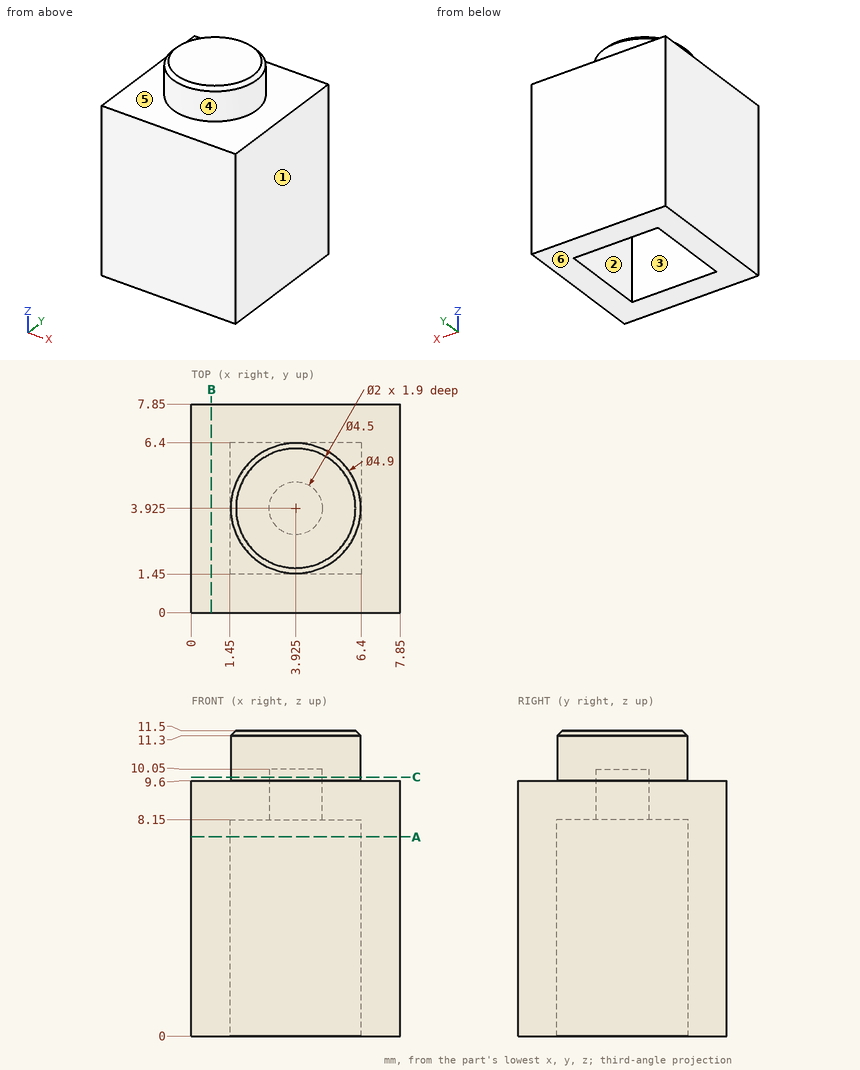
For this review, use the dimensioned drawing (mm, ordinates from the lowest corner) and the shaded views. A direction names the side the tool comes from. Coordinates: 2 decimals unless noted, no trailing zeros. Order: outer loops, then holes, each group sorted by start corner. A loop starts at its lowest first (then second) coordinate and runs counter-clockwise, first axis right, second up. Notation, with made-up numbers: M 52.25,75 L 91.25,75 A21 cw 91.25,112 Z; hole C -18,-34 d3. An arc over 180 degrees is marked long. Answer as a JSON object with one key per item and string values. Group by question number.
1) For pin 1 (1.8 mm diameter, centred on x = 3.925, y = 3.925, fed in from -Z); pin 2 (1.6 mm diameter, centred on x = 4.5, y = 4, fed in from -Z), all flat-tipped, find the tip position at first contact; note any pin that passes through.
2) Add section A-A, the plane z = 7.5. Write out the cut boundary in (x, y), then the cut area to 3 significant figures.
3) Wall thickness on L1, parallel to X at y = 1.5, z = 7.25; L2, parallel to X at y = 4, z = 8.25: over which ranges is each line inside the solid? List them lowest first.
4) Add section B-B, the plane x = 0.75. Write out the cut boundary in (y, z), then the cut area to 3 significant figures.
5) Tool access review of the marked faces 5 and 6: name each direction out of +Z, -Z, +X, -X, +Y, -Y from which nothing blocks a thin tool from reaching the whole face with its end or side.
6) Mouldability with a two-part tool opening along Y and no side actions: class the marked faces 1, 2, 3 and 4 as pulls with the +Y half, pulls with the -Y half, needs draft (parallel to the pull), parting line crosses it, or undercut.
7) Add section C-C, the plane z = 9.75. Write out the cut boundary in (x, y) (3 decimals).
Computed values:
{
 "1": {"pin 1": "stops at z = 10.05", "pin 2": "stops at z = 8.15"},
 "2": {"outline": "M 0,0 L 7.85,0 L 7.85,7.85 L 0,7.85 Z; hole M 1.45,1.45 L 6.4,1.45 L 6.4,6.4 L 1.45,6.4 Z", "area": "37.1 mm^2"},
 "3": {"L1": "x = 0 to 1.45, 6.4 to 7.85", "L2": "x = 0 to 2.93, 4.92 to 7.85"},
 "4": {"outline": "M 0,0 L 7.85,0 L 7.85,9.6 L 0,9.6 Z", "area": "75.4 mm^2"},
 "5": {"face 5": "+Z", "face 6": "-Z, +X, -X, +Y, -Y"},
 "6": {"face 1": "needs draft", "face 2": "undercut", "face 3": "undercut", "face 4": "parting line crosses it"},
 "7": {"outline": "C 3.925,3.925 d4.9; hole C 3.925,3.925 d2"}
}
